Work out the finished part from the listing and answer in its coordinate system (mm). A direction names the side the tool comes from. Coordinates: 2 decimals unless noted, no trailing zeros. Order: outer loops, then holes, each group sorted by start corner. A loop starts at its lowest first (then second) coordinate and runs counter-clockwise, first axis right, second up. Notation, with made-up numbers: M 5.25,-28.75 L 13.25,-28.75 A18 cw 13.25,-19.75 Z; hole C -40,29.25 d3. An arc over 180 degrees is marked long. Use a Markdown table: item, result.
from build123d import *

# Parameters (mm, degrees)
BOSS_EXTRUDE1_DEPTH        = 12.7
CHAMFER1_SIZE              = 2.54
HOLE1_D                    = 4.9784
HOLE2_D                    = 4.9784
F_6_4_6_4_DIAMETER_HOLE1_D = 6.4
FILLET1_START              = -1
FILLET1_DEPTH              = 15
FILLET1_2_DEPTH            = 12.7


with BuildPart() as part:
    # Sketch1 → Boss-Extrude1 (new body)
    with BuildSketch(Plane(origin=(0, 0, 0), x_dir=(-1, 0, 0), z_dir=(0, 0, -1))):
        Polygon((-6.985, 10.668), (-22.225, 10.668), (-22.225, 0), (22.225, 0), (22.225, 10.668), (6.985, 10.668), (6.985, 17.018), (-6.985, 17.018), align=None)
    extrude(amount=-BOSS_EXTRUDE1_DEPTH)

    # Chamfer1
    chamfer1_edges = [part.edges().sort_by_distance(p)[0] for p in [
        (22.225, 5.334, 0),
        (22.225, 5.334, 12.7),
        (-22.225, 5.334, 12.7),
        (-22.225, 5.334, 0),
    ]]
    chamfer(chamfer1_edges, length=CHAMFER1_SIZE)

    # Hole1 (through all)
    with Locations(Plane(origin=(0, 10.668, 0), x_dir=(1, 0, 0), z_dir=(0, 1, 0))):
        with Locations((15.875, -6.35)):
            Hole(HOLE1_D / 2)

    # Hole2 (through all)
    with Locations(Plane(origin=(0, 10.668, 0), x_dir=(1, 0, 0), z_dir=(0, 1, 0))):
        with Locations((-15.875, -6.35)):
            Hole(HOLE2_D / 2)

    # Ø6.4 (6.4) Diameter Hole1 (through all)
    with Locations(Plane.XY.offset(12.7)):
        with Locations((0, 10.668)):
            Hole(F_6_4_6_4_DIAMETER_HOLE1_D / 2)

    # Fillet1: read off the stored shape, not the designer's step
    # Fillet1 outline → Fillet1 (cut)
    with BuildSketch(Plane.XY.offset(FILLET1_START)):
        with BuildLine():
            Line((-6.985, 17.018), (-6.985, 13.843))
            ThreePointArc((-6.985, 13.843), (-6.05506403, 16.08806403), (-3.81, 17.018))
            Line((-3.81, 17.018), (-6.985, 17.018))
        make_face()
        with BuildLine():
            Line((6.985, 17.018), (3.81, 17.018))
            ThreePointArc((3.81, 17.018), (6.05506403, 16.08806403), (6.985, 13.843))
            Line((6.985, 13.843), (6.985, 17.018))
        make_face()
    extrude(amount=FILLET1_DEPTH, mode=Mode.SUBTRACT)

    # Fillet1 2 outline → Fillet1 2 (add)
    with BuildSketch(Plane.XY):
        with BuildLine():
            Line((-6.985, 10.668), (-6.985, 13.843))
            ThreePointArc((-6.985, 13.843), (-7.91493597, 11.59793597), (-10.16, 10.668))
            Line((-10.16, 10.668), (-6.985, 10.668))
        make_face()
        with BuildLine():
            ThreePointArc((10.16, 10.668), (7.91493597, 11.59793597), (6.985, 13.843))
            Line((6.985, 13.843), (6.985, 10.668))
            Line((6.985, 10.668), (10.16, 10.668))
        make_face()
    extrude(amount=FILLET1_2_DEPTH)


solid = part.part
1. For a pull along Z with two mould halves and no side action, classify faces 1 (the face through (0, 0, 6)), 2 (the face through (18.36, 5.26, 6.24)), 3 (the face through (-20.937, 5.259, 1.252)) as +Z half, -Z half, draft (parallel to the pull), parting line (faces both ways), or undercut.
Answers below:
| item | result |
|---|---|
| face 1 | draft |
| face 2 | undercut |
| face 3 | -Z half |
2. Section B-B on z = 6.35 is taken. Determine the outline of the cut face in (x, y) (3 decimals), then the cut area to 3 significant figures.
Answers below:
| item | result |
|---|---|
| outline | M -22.225,0 L -18.364,0 L -18.364,10.668 L -22.225,10.668 Z; M -13.386,0 L 13.386,0 L 13.386,10.668 L 10.16,10.668 A3.175 cw 6.985,13.843 A3.175 ccw 3.81,17.018 L -3.81,17.018 A3.175 ccw -6.985,13.843 A3.175 cw -10.16,10.668 L -13.386,10.668 Z; M 18.364,0 L 22.225,0 L 22.225,10.668 L 18.364,10.668 Z; hole C 0,10.668 d6.4 |
| area | 425 mm² |
3. A flat-ended cylindrical pin translates along its axis: P1, Ø2, axis at x = 10.5, z = 2, coming from the +Y side. Find the tip coordinate at first contact, or state that the pin passes through.
Answers below:
| item | result |
|---|---|
| P1 | y = 10.74 |
4. Section A-A on x = 0 is taken. Determine the outline of the cut face in (y, z), then the cut area to 3 significant figures.
Answers below:
| item | result |
|---|---|
| outline | M 0,0 L 7.47,0 L 7.47,12.7 L 0,12.7 Z; M 13.87,0 L 17.02,0 L 17.02,12.7 L 13.87,12.7 Z |
| area | 135 mm² |
5. For faces 4 (the face through (-19, 10.668, 6)), 5 (the face through (19, 10.668, 6)), 6 (the face through (20.937, 5.409, 11.448)), determine the directions among +Z, -Z, +X, -X, +Y, -Y from which every point of the face is accessible in a straight line to the end or side of a thin tool.
Answers below:
| item | result |
|---|---|
| face 4 | +Z, -Z, -X, +Y |
| face 5 | +Z, -Z, +X, +Y |
| face 6 | +Z, +X, +Y, -Y |
6. Section D-D on y = 4.25 is taken. Determine the outline of the cut face in (x, z) (3 decimals).
Answers below:
| item | result |
|---|---|
| outline | M -22.225,2.54 L -19.685,0 L 19.685,0 L 22.225,2.54 L 22.225,10.16 L 19.685,12.7 L -19.685,12.7 L -22.225,10.16 Z; hole C -15.875,6.35 d4.978; hole C 15.875,6.35 d4.978 |
7. Find the intervals of material crossed by probe 1 along X at (y, z) = (4.5, 6.5) (3 decimals); probe 2 along Y at (x, z) = (0, 9.25); probe 3 along X at (y, z) = (9.5, 2.5) (3 decimals), in increasing order.
Answers below:
| item | result |
|---|---|
| probe 1 | -22.225 to -18.36, -13.39 to 13.39, 18.36 to 22.225 |
| probe 2 | 0 to 7.47, 13.87 to 17.02 |
| probe 3 | -22.185 to -2.979, 2.979 to 22.185 |
8. Section C-C on y = 10.25 is taken. Determine the outline of the cut face in (x, z) (3 decimals).
Answers below:
| item | result |
|---|---|
| outline | M -22.225,2.54 L -19.685,0 L -3.173,0 L -3.173,12.7 L -19.685,12.7 L -22.225,10.16 Z; M 3.173,0 L 19.685,0 L 22.225,2.54 L 22.225,10.16 L 19.685,12.7 L 3.173,12.7 Z; hole C -15.875,6.35 d4.978; hole C 15.875,6.35 d4.978 |
